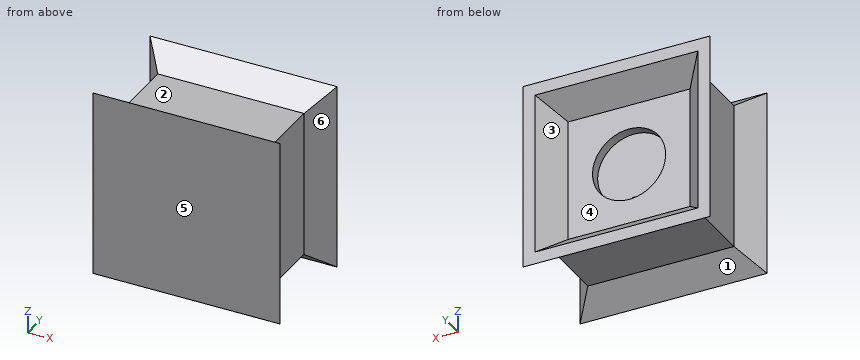
```python
from build123d import *

# Parameters (mm, degrees)
SKETCH1_W               = 76.2
SKETCH1_H               = 76.2
BOSS_EXTRUDE1_DEPTH     = 15.875
SKETCH2_W               = 76.2
SKETCH2_H               = 76.2
BOSS_EXTRUDE2_DEPTH     = 12.7
BOSS_EXTRUDE2_DRAFT     = -40
MIRROR1_COPY_1_SKETCH_W = 76.2
MIRROR1_COPY_1_SKETCH_H = 76.2
MIRROR1_COPY_1_DEPTH    = 12.7
MIRROR1_COPY_1_DRAFT    = -40
SKETCH4_W               = 84.813130632
SKETCH4_H               = 84.813130632
CUT_EXTRUDE2_DEPTH      = 12.7
CUT_EXTRUDE2_DRAFT      = -40
SKETCH5_R               = 19.05
CUT_EXTRUDE3_DEPTH      = 5.08
SKETCH6_R               = 1.524
CUT_EXTRUDE4_DEPTH      = 20.32


with BuildPart() as part:
    # Sketch1 → Boss-Extrude1 (new, symmetric)
    with BuildSketch(Plane(origin=(0, 0, 0), x_dir=(1, 0, 0), z_dir=(0, 1, 0))):
        Rectangle(SKETCH1_W, SKETCH1_H)
    extrude(amount=BOSS_EXTRUDE1_DEPTH, both=True)


with BuildPart() as boss_extrude2_tool:
    # Sketch2 → Boss-Extrude2 (with draft: the straight prism first)
    with BuildSketch(Plane(origin=(0, 15.875, 0), x_dir=(1, 0, 0), z_dir=(0, 1, 0))):
        Rectangle(SKETCH2_W, SKETCH2_H)
    extrude(amount=BOSS_EXTRUDE2_DEPTH)
    # Boss-Extrude2: the draft: its side faces are tilted about the plane it starts from
    boss_extrude2_sides = [boss_extrude2_tool.faces().sort_by_distance(p)[0] for p in [
        (-38.1, 22.225, 0),
        (0, 22.225, 38.1),
        (38.1, 22.225, 0),
        (0, 22.225, -38.1),
    ]]
    draft(boss_extrude2_sides, Plane(origin=(0, 15.875, 0), x_dir=(1, 0, 0), z_dir=(0, 1, 0)), BOSS_EXTRUDE2_DRAFT)


with BuildPart() as part_1:
    add(part.part)

    # Boss-Extrude2: add boss_extrude2_tool
    add(boss_extrude2_tool.part)


with BuildPart() as mirror1_copy_1_tool:
    # Mirror1 copy 1 sketch → Mirror1 copy 1 (with draft: the straight prism first)
    with BuildSketch(Plane.XZ.offset(15.875)):
        Rectangle(MIRROR1_COPY_1_SKETCH_W, MIRROR1_COPY_1_SKETCH_H)
    extrude(amount=MIRROR1_COPY_1_DEPTH)
    # Mirror1 copy 1: the draft: its side faces are tilted about the plane it starts from
    mirror1_copy_1_sides = [mirror1_copy_1_tool.faces().sort_by_distance(p)[0] for p in [
        (-38.1, -22.225, 0),
        (0, -22.225, 38.1),
        (38.1, -22.225, 0),
        (0, -22.225, -38.1),
    ]]
    draft(mirror1_copy_1_sides, Plane.XZ.offset(15.875), MIRROR1_COPY_1_DRAFT)


with BuildPart() as part_2:
    add(part_1.part)

    # Mirror1 copy 1: add mirror1_copy_1_tool
    add(mirror1_copy_1_tool.part)


with BuildPart() as cut_extrude2_tool:
    # Sketch4 → Cut-Extrude2 (with draft: the straight prism first)
    with BuildSketch(Plane(origin=(0, 28.575, 0), x_dir=(1, 0, 0), z_dir=(0, 1, 0))):
        Rectangle(SKETCH4_W, SKETCH4_H)
    extrude(amount=-CUT_EXTRUDE2_DEPTH)
    # Cut-Extrude2: the draft: its side faces are tilted about the plane it starts from
    cut_extrude2_sides = [cut_extrude2_tool.faces().sort_by_distance(p)[0] for p in [
        (42.406565316, 22.225, 0),
        (0, 22.225, -42.406565316),
        (-42.406565316, 22.225, 0),
        (0, 22.225, 42.406565316),
    ]]
    draft(cut_extrude2_sides, Plane(origin=(0, 28.575, 0), x_dir=(1, 0, 0), z_dir=(0, 1, 0)), CUT_EXTRUDE2_DRAFT)


with BuildPart() as part_3:
    add(part_2.part)

    # Cut-Extrude2: cut by cut_extrude2_tool
    add(cut_extrude2_tool.part, mode=Mode.SUBTRACT)

    # Sketch5 → Cut-Extrude3 (cut)
    with BuildSketch(Plane(origin=(0, 15.875, 0), x_dir=(1, 0, 0), z_dir=(0, 1, 0))):
        with Locations(Location((0, 0, 0), (0, 0, 270))):
            Circle(SKETCH5_R)
    extrude(amount=-CUT_EXTRUDE3_DEPTH, mode=Mode.SUBTRACT)

    # Sketch6 → Cut-Extrude4 (cut)
    with BuildSketch(Plane(origin=(0, 10.795, 0), x_dir=(1, 0, 0), z_dir=(0, 1, 0))):
        with Locations(Location((0, 16.51, 0), (0, 0, 270))):
            Circle(SKETCH6_R)
    extrude(amount=-CUT_EXTRUDE4_DEPTH, mode=Mode.SUBTRACT)


solid = part_3.part
```
Model file for the job. Use its own axes, mm. Face numbers are marked on the shaded views. A direction names the side the tool comes from. Coordinates: 2 decimals unless noted, no trailing zeros. Order: outer loops, then holes, each group sorted by start corner. A loop starts at its lowest first (then second) coordinate and runs counter-clockwise, first axis right, second up. Notation, with made-up numbers: M 25,2.25 L 41,2.25 A32 ccw 41,40.25 Z; hole C -32.75,35 d8. An arc over 180 degrees is marked long. Answer as CSV lines item,"result".
(1) Band-saw the part on C-C, the plane y = -6.5. List the corners of the cut face in (x, z), then the cut area to 3 significant figures.
Geometry says:
outline,"M -38.1,-38.1 L 38.1,-38.1 L 38.1,38.1 L -38.1,38.1 Z; hole C 0,-16.51 d3.05"
area,"5,800 mm2"
(2) Band-saw the part on A-A, the plane x = 0. List the corners of the cut face in (y, z) (3 decimals), then the cut area to 3 significant figures.
Geometry says:
outline,"M -28.575,-48.757 L -15.875,-38.1 L 15.875,-38.1 L 28.575,-48.757 L 28.575,-42.407 L 15.875,-31.75 L 15.875,-19.05 L 10.795,-19.05 L 10.795,-18.034 L -9.525,-18.034 L -9.525,-14.986 L 10.795,-14.986 L 10.795,19.05 L 15.875,19.05 L 15.875,31.75 L 28.575,42.407 L 28.575,48.757 L 15.875,38.1 L -15.875,38.1 L -28.575,48.757 Z"
area,"3,430 mm2"
(3) Flat gauge pins, fed straight in: pin 1 (1 mm diameter, centred on x = 28, z = 21.5, fed in from +Y) (3 decimals); pin 2 (5 mm diameter, centred on x = -16, z = -38, fed in from +Y); pin 3 (9.5 mm diameter, centred on x = 2.5, y = 7.5, fed in from -Z). Where does each tip first touch, or does it go through?
Geometry says:
pin 1,"stops at y = 15.875"
pin 2,"stops at y = 26.3"
pin 3,"stops at z = -38.1"
(4) 3-axis set-ups, long thin cutter, end or side, ignore diameter. For the marked faces 1, 2 and 3: which of +Z, -Z, +X, -X, +Y, -Y reach the whole face in a straight line?
Geometry says:
face 1,"-Z, +X, -X"
face 2,"+Z, +X, -X"
face 3,"+Y"
(5) Band-saw the part on D-D, the plane z = -16.51. List the corners of the cut face in (x, y) (3 decimals).
Geometry says:
outline,"M -48.757,-28.575 L 48.757,-28.575 L 38.1,-15.875 L 38.1,15.875 L 48.757,28.575 L 42.407,28.575 L 31.75,15.875 L 9.504,15.875 L 9.504,10.795 L 1.524,10.795 L 1.524,-9.525 L -1.524,-9.525 L -1.524,10.795 L -9.504,10.795 L -9.504,15.875 L -31.75,15.875 L -42.407,28.575 L -48.757,28.575 L -38.1,15.875 L -38.1,-15.875 Z"
(6) Pull direction Y, two halves, no side cores. Call the marked faces 4, 5 and 6: +Y half, -Y half, draft (parallel to the pull), parting line (faces both ways), or undercut.
Geometry says:
face 4,"+Y half"
face 5,"-Y half"
face 6,"undercut"
(7) Band-saw the part on B-B, the plane z = 0. List the corners of the cut face in (x, y) (3 decimals), then the cut area to 3 significant figures.
Geometry says:
outline,"M -48.757,-28.575 L 48.757,-28.575 L 38.1,-15.875 L 38.1,15.875 L 48.757,28.575 L 42.407,28.575 L 31.75,15.875 L 19.05,15.875 L 19.05,10.795 L -19.05,10.795 L -19.05,15.875 L -31.75,15.875 L -42.407,28.575 L -48.757,28.575 L -38.1,15.875 L -38.1,-15.875 Z"
area,"3,490 mm2"
(8) Wall check: line 1 along X through (y, z) = (-1.75, -16.51); line 2 along Y through (x, z) = (30, -24) (3 decimals); line 3 along Z through (x, y) = (-6.5, -10.5). Give the ranges that are in metal, low to high.
Geometry says:
line 1,"x = -38.1 to -1.52, 1.52 to 38.1"
line 2,"y = -28.575 to 15.875"
line 3,"z = -38.1 to 38.1"
